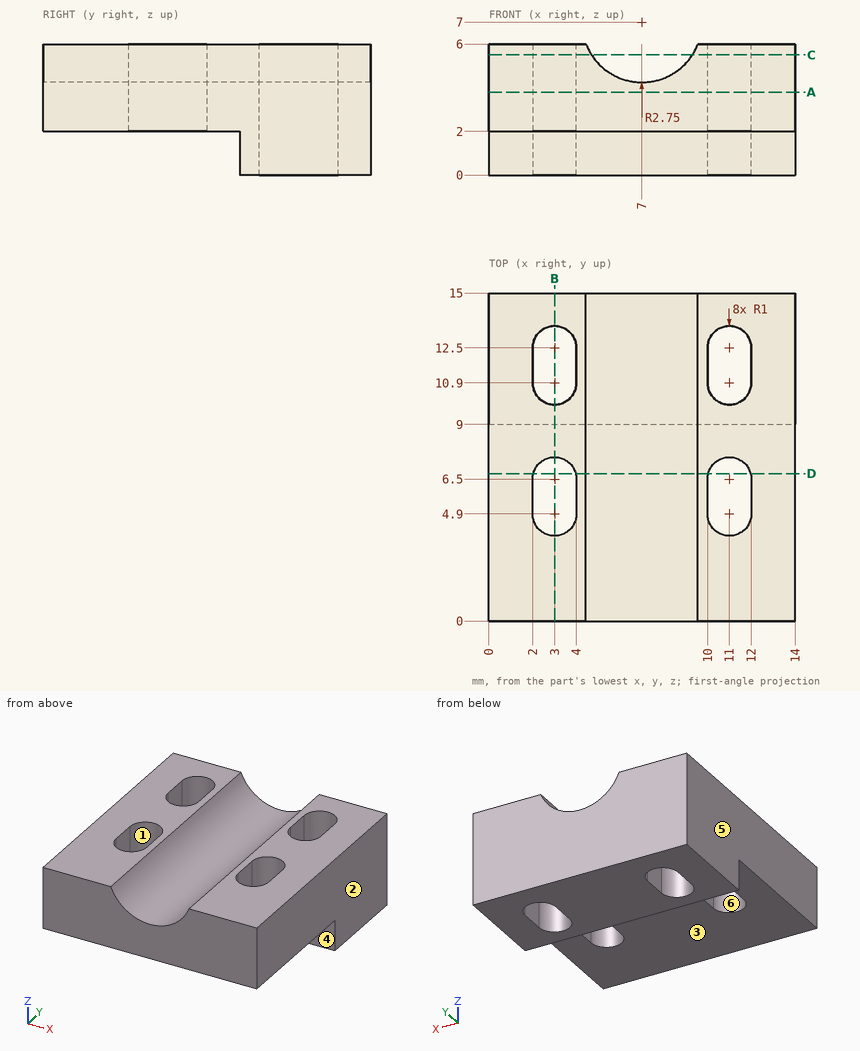
Source: three-view drawing plus pictorial views. Frame: mm from the lowest corner of the part. A direction names the side the tool comes from. Give positions to 0.01 mm unless a question says otherwise; leave off trailing zeros. Write each loop counter-clockwise with the first axis right and the second up, starting at its lowest first coordinate (ties: lowest second). Pieces come first, ordered by that corner, then holes. Notation, with made-up numbers: (-33.5, -19.5) -> (18.5, -19.5) arc R20 cw to (18.5, -13.5) -> close; hole circle Ø5 at (69, 64.25). An arc over 180 degrees is marked (long way). Answer in a Markdown table with one row per item.
(1) Section query D-D on y = 6.75. Return loops of the section in (x, z), then the cut area to 3 significant figures.
Answers below:
| item | result |
|---|---|
| outline | (0, 2) -> (2.03, 2) -> (2.03, 6) -> (0, 6) -> close; (3.97, 2) -> (10.03, 2) -> (10.03, 6) -> (9.56, 6) arc R2.75 cw to (4.44, 6) -> (3.97, 6) -> close; (11.97, 2) -> (14, 2) -> (14, 6) -> (11.97, 6) -> close |
| area | 34.0 mm^2 |
(2) Ray query, line 1 along X through (y, z) = (12, 1.35); line 2 along Y through (x, z) = (0.5, 1.7); line 3 along Y through (x, z) = (2.5, 1.85). Return the intervals inside material, ascending. Write a range as [from, to].
Answers below:
| item | result |
|---|---|
| line 1 | [0, 2], [4, 10], [12, 14] |
| line 2 | [9, 15] |
| line 3 | [9, 10.03], [13.37, 15] |
(3) Set-up query: the marked faces 1, 2 and 3. Return all of +Z, -Z, +X, -X, +Y, -Y with unobstructed straight access to the full face (end or side cutting, diameter ignored); none if empty.
Answers below:
| item | result |
|---|---|
| face 1 | +Z, -Z |
| face 2 | +Z, -Z, +X, +Y, -Y |
| face 3 | -Z, +X, -X, -Y |
(4) Draft query along X for the marked faces 4, 5 and 6. Return one class per face: +X half, -X half, draft (parallel to the pull), parting line (faces both ways), or undercut.
Answers below:
| item | result |
|---|---|
| face 4 | draft |
| face 5 | -X half |
| face 6 | undercut |
(5) Pin query (flat end, axial travel): pin 1 (1.6 mm diameter, centred on x = 5, z = 1, fed in from -Y). Return the tip coordinate at first contact, or that it passes through.
Answers below:
| item | result |
|---|---|
| pin 1 | y = 9 |
(6) Section query A-A on z = 3.8. Return loops of the section in (x, y), then the cut area to 3 significant figures.
Answers below:
| item | result |
|---|---|
| outline | (0, 0) -> (14, 0) -> (14, 15) -> (0, 15) -> close; hole (2, 4.9) arc R1 ccw to (4, 4.9) -> (4, 6.5) arc R1 ccw to (2, 6.5) -> close; hole (2, 10.9) arc R1 ccw to (4, 10.9) -> (4, 12.5) arc R1 ccw to (2, 12.5) -> close; hole (10, 4.9) arc R1 ccw to (12, 4.9) -> (12, 6.5) arc R1 ccw to (10, 6.5) -> close; hole (10, 10.9) arc R1 ccw to (12, 10.9) -> (12, 12.5) arc R1 ccw to (10, 12.5) -> close |
| area | 185 mm^2 |
(7) Section query B-B on x = 3. Return loops of the section in (y, z), then the cut area to 3 significant figures.
Answers below:
| item | result |
|---|---|
| outline | (0, 2) -> (3.9, 2) -> (3.9, 6) -> (0, 6) -> close; (7.5, 2) -> (9, 2) -> (9, 0) -> (9.9, 0) -> (9.9, 6) -> (7.5, 6) -> close; (13.5, 0) -> (15, 0) -> (15, 6) -> (13.5, 6) -> close |
| area | 36.0 mm^2 |
(8) Section query C-C on z = 5.5. Return loops of the section in (x, y).
Answers below:
| item | result |
|---|---|
| outline | (0, 0) -> (4.7, 0) -> (4.7, 15) -> (0, 15) -> close; (9.3, 0) -> (14, 0) -> (14, 15) -> (9.3, 15) -> close; hole (2, 4.9) arc R1 ccw to (4, 4.9) -> (4, 6.5) arc R1 ccw to (2, 6.5) -> close; hole (2, 10.9) arc R1 ccw to (4, 10.9) -> (4, 12.5) arc R1 ccw to (2, 12.5) -> close; hole (10, 4.9) arc R1 ccw to (12, 4.9) -> (12, 6.5) arc R1 ccw to (10, 6.5) -> close; hole (10, 10.9) arc R1 ccw to (12, 10.9) -> (12, 12.5) arc R1 ccw to (10, 12.5) -> close |
